Check sheet for the modelled part. Datum: model origin and axes. Units: mm. A direction names the side the tool comes from. Give positions to 0.01 mm unless a question says otherwise; leave off trailing zeros. Write each loop counter-clockwise with the first axis right and the second up, starting at its lowest first coordinate (ties: lowest second). Pieces come first, ordered by that corner, then holes. Notation, with made-up numbers: M 64,-26.75 L 73,-26.75 A28 ccw 73,1.25 Z; hole C 68.25,7 d3. An arc over 180 degrees is marked long. Write item = value, one per line. Start each with the question number.
1) Set-up check for faces 5 (the face through (12.7, 32, 2)), 6 (the face through (0, 31, 2)), 7 (the face through (38.1, 8, 2)): record each of +Z, -Z, +X, -X, +Y, -Y from which the full face is reachable in a straight line by a thin tool's end or side.
2) Scan lines: L1, parallel to Y at x = -25.4, z = 1.45; L2, parallel to Y at x = -18, z = 4.05; L3, parallel to X at y = 8, z = 0.7. Record each from-to range of solid material in increasing order.
3) Gauge pin test, flat end, axial feed: pin 1 (1.5 mm diameter, centred on y = 27, z = 2.5, fed in from +X). Record the tip position at first contact, or that the pin passes through.
4) Draft check along Y on faces 1 (the face through (-34, -25.4, 2)), 2 (the face through (28.173, 6.362, 2.348)), 3 (the face through (-26.63, 81.74, 2.35)), 4 (the face through (28.93, 80.21, 2.35)). Enter one of: pulls with the +Y half, pulls with the -Y half, needs draft (parallel to the pull), parting line crosses it, or undercut.
5) Sectioned sample at D-D, the plane x = 16. Record the cut outline in (y, z), then the cut area to 3 significant figures.
6) Sectioned sample at C-C, the plane y = 33. Record the cut outline in (x, z).
7) Sectioned sample at A-A, the plane x = -32. Record the cut outline in (y, z).
8) Sectioned sample at B-B, the plane z = 3.75. Count the separate pieces of the cut face and the enclosed holes in it, then the cut area to 3 significant figures.
from build123d import *

# Parameters (mm, degrees)
SKETCH1_R           = 2.286
SKETCH1_R_2         = 2.667
BOSS_EXTRUDE1_DEPTH = 4.7625


with BuildPart() as part:
    # Sketch1 → Boss-Extrude1 (new body)
    with BuildSketch(Plane.XY):
        with BuildLine():
            Line((0, 0), (0, 63.5))
            Line((0, 63.5), (-76.2, 63.5))
            Line((-76.2, 63.5), (-76.2, 88.9))
            Line((-76.2, 88.9), (7.62, 88.9))
            ThreePointArc((7.62, 88.9), (29.172614691, 79.972614691), (38.1, 58.42))
            Line((38.1, 58.42), (38.1, 52.197))
            Line((38.1, 52.197), (12.7, 52.197))
            Line((12.7, 52.197), (12.7, 11.303))
            Line((12.7, 11.303), (38.1, 11.303))
            Line((38.1, 11.303), (38.1, 5.08))
            ThreePointArc((38.1, 5.08), (29.172614691, -16.472614691), (7.62, -25.4))
            Line((7.62, -25.4), (-76.2, -25.4))
            Line((-76.2, -25.4), (-76.2, 0))
            Line((-76.2, 0), (0, 0))
        make_face()
        with Locations(Location((20.447, 56.4515, 0), (0, 0, 180))):
            Circle(SKETCH1_R, mode=Mode.SUBTRACT)
        with Locations(Location((30.353, 56.4515, 0), (0, 0, 180))):
            Circle(SKETCH1_R, mode=Mode.SUBTRACT)
        with Locations(Location((20.447, 7.0485, 0), (0, 0, 180))):
            Circle(SKETCH1_R, mode=Mode.SUBTRACT)
        with Locations(Location((30.353, 7.0485, 0), (0, 0, 180))):
            Circle(SKETCH1_R, mode=Mode.SUBTRACT)
        with Locations(Location((-50.8, 79.375, 0), (0, 0, 180))):
            Circle(SKETCH1_R_2, mode=Mode.SUBTRACT)
        with Locations(Location((-25.4, 79.375, 0), (0, 0, 180))):
            Circle(SKETCH1_R_2, mode=Mode.SUBTRACT)
        with Locations(Location((-50.8, -15.875, 0), (0, 0, 180))):
            Circle(SKETCH1_R_2, mode=Mode.SUBTRACT)
        with Locations(Location((-25.4, -15.875, 0), (0, 0, 180))):
            Circle(SKETCH1_R_2, mode=Mode.SUBTRACT)
    extrude(amount=BOSS_EXTRUDE1_DEPTH)


solid = part.part
Data:
q1.face_5 = +Z, -Z, +X
q1.face_6 = +Z, -Z, -X
q1.face_7 = +Z, -Z, +X, +Y, -Y
q2.L1 = -25.4 to -18.54, -13.21 to 0, 63.5 to 76.71, 82.04 to 88.9
q2.L2 = -25.4 to 0, 63.5 to 88.9
q2.L3 = 0 to 18.37, 22.53 to 28.27, 32.43 to 38.1
q3.pin_1 = 12.7
q4.face_1 = pulls with the -Y half
q4.face_2 = undercut
q4.face_3 = undercut
q4.face_4 = pulls with the +Y half
q5.outline = M -24.23,0 L 11.3,0 L 11.3,4.76 L -24.23,4.76 Z; M 52.2,0 L 87.73,0 L 87.73,4.76 L 52.2,4.76 Z
q5.area = 338 mm2
q6.outline = M 0,0 L 12.7,0 L 12.7,4.76 L 0,4.76 Z
q7.outline = M -25.4,0 L 0,0 L 0,4.76 L -25.4,4.76 Z; M 63.5,0 L 88.9,0 L 88.9,4.76 L 63.5,4.76 Z
q8.separate_pieces = 1
q8.enclosed_holes = 8
q8.area = 6,630 mm2
